Model file for the job. Use its own axes, mm. Face numbers are marked on the shaded views. A direction names the side the tool comes from. Coordinates: 2 decimals unless noted, no trailing zeros. Write each loop counter-clockwise with the first axis right and the second up, starting at its lowest first coordinate (ties: lowest second). Pieces come first, ordered by that corner, then holes. Notation, with made-up numbers: (3, 3.5) - (47, 3.5) arc R23 cw to (47, 38.5) - close; hole circle Ø9 at (-29, 81.5). An arc over 180 degrees is marked (long way). Put each result on its own line as item: value. Start each with the question number.
1. Saw through at C-C, the plane x = -15. Write the cut outline in (y, z).
2. Saw through at B-B, the plane z = 19.05. Write the cut outline in (x, y).
3. Drill centre lines: L1, parallel to Z at x = 30.75, y = 6.35; L2, parallel to Z at x = 12.5, y = 9.25; L3, parallel to Y at x = 22.5, z = -19.05. Where is each one in solid material? Low to high. Write a range as from..to.
4. Saw through at D-D, the plane y = 7.25. Give the number of separate pieces and of enclosed holes in the cut face, plus the area to 3 significant figures.
5. Which spindle directions (+Z, -Z, +X, -X, +Y, -Y) get a long thin tool onto all of the face, cutting with end or side? Do the marked faces 4, 5 and 6. Say none if no direction does.
6. Pull direction Z, two halves, no side cores. Call the marked faces 1, 2 and 3: released by +Z, released by -Z, zero draft, split by the parting line, or undercut.
7. Drop flat-ended pins along their axis: P1, Ø5.5, axis at y = 3, z = 22, coming from the -X side; P2, Ø4, axis at x = -1, y = 9, coming from the +Z side; P3, Ø6.5, axis at x = -4, y = 8, coming from the -Z side; P4, Ø6, axis at y = 6.35, z = -19.05, coming from the +X side. Give the stop position or say it passes through.
8. Saw through at A-A, the plane x = 24.5. Write the cut outline in (y, z).
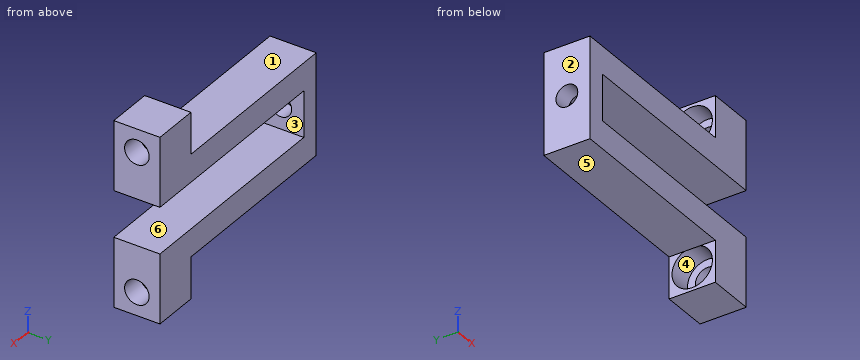
```python
from build123d import *

# Parameters (mm, degrees)
SKETCH1_W                                     = 64.2
SKETCH1_H                                     = 50.8
BOSS_EXTRUDE1_DEPTH                           = 12.7
SKETCH4_W                                     = 51.5
SKETCH4_H                                     = 11.43
SKETCH4_W_2                                   = 59.12
SKETCH4_H_2                                   = 12.7
CUT_EXTRUDE1_DEPTH                            = 12.7
CBORE_FOR_1_4_SOCKET_HEAD_CAP_SCREW1_AT_COUNT = 2
CBORE_FOR_1_4_SOCKET_HEAD_CAP_SCREW1_AT_PITCH = 38.1
F_6_0MM_DOWEL_HOLE1_D                         = 6


with BuildPart() as part:
    # Sketch1 → Boss-Extrude1 (new body)
    with BuildSketch(Plane(origin=(0, 0, 0), x_dir=(1, 0, 0), z_dir=(0, 1, 0))):
        Rectangle(SKETCH1_W, SKETCH1_H)
    extrude(amount=BOSS_EXTRUDE1_DEPTH)

    # Sketch4 → Cut-Extrude1 (cut)
    with BuildSketch(Plane(origin=(0, 12.7, 0), x_dir=(1, 0, 0), z_dir=(0, 1, 0))):
        with Locations((-6.35, -19.685)):
            Rectangle(SKETCH4_W, SKETCH4_H)
        with Locations((-6.35, 19.685)):
            Rectangle(SKETCH4_W, SKETCH4_H)
        with Locations((2.54, 0)):
            Rectangle(SKETCH4_W_2, SKETCH4_H_2)
    extrude(amount=-CUT_EXTRUDE1_DEPTH, mode=Mode.SUBTRACT)

    # Sketch6 → CBORE for 1/4 Socket Head Cap Screw1 (revolve, cut)
    with BuildSketch(Plane(origin=(19.4, 6.35, 19.05), x_dir=(0, 0, 1), z_dir=(0, 1, 0))):
        Polygon((0, 0), (0, 12.7), (3.3782, 12.7), (3.3782, 6.35), (5.55625, 6.35), (5.55625, 0), align=None)
    cbore_for_1_4_socket_head_cap_screw1 = revolve(axis=Axis((13.05, 6.35, 19.05), (1, 0, 0)), mode=Mode.SUBTRACT)

    # CBORE for 1/4 Socket Head Cap Screw1 at: CBORE for 1/4 Socket Head Cap Screw1 ×2
    with Locations(*[(0, 0, -i * CBORE_FOR_1_4_SOCKET_HEAD_CAP_SCREW1_AT_PITCH) for i in range(1, CBORE_FOR_1_4_SOCKET_HEAD_CAP_SCREW1_AT_COUNT)]):
        add(cbore_for_1_4_socket_head_cap_screw1, mode=Mode.SUBTRACT)

    # Ø6.0mm Dowel Hole1 (through all)
    with Locations(Plane.ZY.offset(32.1)):
        with Locations((0, 6.35)):
            Hole(F_6_0MM_DOWEL_HOLE1_D / 2)


solid = part.part
```
Final values:
1. outline: (0, -13.97) - (12.7, -13.97) - (12.7, -6.35) - (0, -6.35) - close; (0, 6.35) - (12.7, 6.35) - (12.7, 13.97) - (0, 13.97) - close
2. outline: (19.4, 0) - (32.1, 0) - (32.1, 2.97) - (25.75, 2.97) - (25.75, 0.79) - (19.4, 0.79) - close; (19.4, 11.91) - (25.75, 11.91) - (25.75, 9.73) - (32.1, 9.73) - (32.1, 12.7) - (19.4, 12.7) - close
3. L1: z = -25.4..-22.43, -15.67..-6.35, 6.35..15.67, 22.43..25.4
3. L2: z = -13.97..-6.35, 6.35..13.97
3. L3: y = 0..0.79, 11.91..12.7
4. separate pieces: 4
4. enclosed holes: 0
4. area: 1,080 mm²
5. face 4: none
5. face 5: -Z, -X, +Y, -Y
5. face 6: +X, +Y, -Y
6. face 1: released by +Z
6. face 2: zero draft
6. face 3: undercut
7. P1: stops at x = 19.4
7. P2: stops at z = 13.97
7. P3: stops at z = -13.97
7. P4: passes through
8. outline: (0, -25.4) - (12.7, -25.4) - (12.7, -6.35) - (0, -6.35) - close; (0, 6.35) - (12.7, 6.35) - (12.7, 25.4) - (0, 25.4) - close; hole circle Ø11.11 at (6.35, -19.05); hole circle Ø11.11 at (6.35, 19.05)
